from build123d import *

# Parameters (mm, degrees)
F1_DEPTH      = 16.002
F2_R          = 6.1442753349
F2_R_2        = 6.1243758279
F3_DEPTH      = 16.003
F5_DEPTH      = 25.4
F5_DEPTH_BACK = 25.4
F7_DEPTH      = 24.13
F7_DEPTH_BACK = 27.178
F8_R          = 3.5427392295
F9_DEPTH      = 25.4
F9_DEPTH_BACK = 25.4


with BuildPart() as f1:
    # F0 (on Top) → F1 (new body)
    with BuildSketch(Plane.XY):
        with BuildLine():
            Line((-13.3363356008, 47.4925674498), (13.3363356008, 47.4925674498))
            ThreePointArc((13.3363356008, 47.4925674498), (0, 60.8289030506), (-13.3363356008, 47.4925674498))
        make_face()
        with BuildLine():
            Line((13.3894772224, 47.4925674498), (13.3363356008, 47.4925674498))
            ThreePointArc((13.3363356008, 47.4925674498), (0, 34.156231849), (-13.3363356008, 47.4925674498))
            Line((-13.3363356008, 47.4925674498), (-13.3363356008, -46.5860655079))
            ThreePointArc((-13.3363356008, -46.5860655079), (0.5964639692, -34.4016239833), (13.3894772224, -47.7778092027))
            Line((13.3894772224, -47.7778092027), (13.3894772224, 47.4925674498))
        make_face()
        with BuildLine():
            ThreePointArc((-13.3363356008, 47.4925674498), (0, 34.156231849), (13.3363356008, 47.4925674498))
            Line((13.3363356008, 47.4925674498), (-13.3363356008, 47.4925674498))
        make_face()
        with BuildLine():
            Line((-13.3363356008, -47.7778092027), (-13.3363356008, -46.5860655079))
            ThreePointArc((-13.3363356008, -46.5860655079), (-0.5964639692, -61.1539944221), (13.3894772224, -47.7778092027))
            Line((13.3894772224, -47.7778092027), (-13.3363356008, -47.7778092027))
        make_face()
        with BuildLine():
            ThreePointArc((13.3894772224, -47.7778092027), (0.5964639692, -34.4016239833), (-13.3363356008, -46.5860655079))
            Line((-13.3363356008, -46.5860655079), (-13.3363356008, -47.7778092027))
            Line((-13.3363356008, -47.7778092027), (13.3894772224, -47.7778092027))
        make_face()
    extrude(amount=F1_DEPTH)

    # F2 (on Top) → F3 (cut, through all)
    with BuildSketch(Plane.XY):
        with Locations((0, 44.9254028499)):
            Circle(F2_R)
        with Locations((0, -46.6368459165)):
            Circle(F2_R_2)
    extrude(amount=F3_DEPTH, mode=Mode.SUBTRACT)

    # F4 (on Front) → F5 (join, two sides)
    with BuildSketch(Plane.XZ) as f5_sk:
        with BuildLine():
            ThreePointArc((6.5605365671, 36.938665784), (6.6343469805, 37.5070254574), (6.6590113547, 38.0796268582))
            ThreePointArc((6.6590113547, 38.0796268582), (0, 44.7386382129), (-6.6590113547, 38.0796268582))
            Line((-6.6590113547, 38.0796268582), (6.5605365671, 38.0796268582))
            Line((6.5605365671, 38.0796268582), (6.5605365671, 36.938665784))
        make_face()
        with BuildLine():
            Line((6.5605365671, 38.0796268582), (-6.6590113547, 38.0796268582))
            ThreePointArc((-6.6590113547, 38.0796268582), (-0.5726014008, 31.4452798778), (6.5605365671, 36.938665784))
            Line((6.5605365671, 36.938665784), (6.5605365671, 38.0796268582))
        make_face()
        with BuildLine():
            ThreePointArc((6.5605365671, 36.938665784), (-0.5726014008, 31.4452798778), (-6.6590113547, 38.0796268582))
            Line((-6.6590113547, 38.0796268582), (-6.6590113547, 2.7097861748))
            Line((-6.6590113547, 2.7097861748), (6.5605365671, 2.7097861748))
            Line((6.5605365671, 2.7097861748), (6.5605365671, 36.938665784))
        make_face()
    extrude(amount=F5_DEPTH)
    extrude(f5_sk.sketch, amount=-F5_DEPTH_BACK)

    # F6 (on Right) → F7 (cut, two sides)
    with BuildSketch(Plane.YZ) as f7_sk:
        with BuildLine():
            Line((6.0519274602, 27.9823391251), (6.0519274602, 27.4877400585))
            ThreePointArc((6.0519274602, 27.4877400585), (6.0557152675, 27.6113640409), (6.0569780455, 27.7350395918))
            ThreePointArc((6.0569780455, 27.7350395918), (6.0557152675, 27.8587151427), (6.0519274602, 27.9823391251))
        make_face()
        with BuildLine():
            Line((-6.0569780165, 27.7344470214), (6.0519274602, 27.4877400585))
            Line((6.0519274602, 27.4877400585), (6.0519274602, 27.9823391251))
            ThreePointArc((6.0519274602, 27.9823391251), (-0.1239717742, 33.7907488023), (-6.0569780165, 27.7344470214))
        make_face()
        with BuildLine():
            ThreePointArc((-6.0569780165, 27.7344470214), (-0.1233793273, 21.6793182817), (6.0519274602, 27.4877400585))
            Line((6.0519274602, 27.4877400585), (-6.0569780165, 27.7344470214))
        make_face()
        with BuildLine():
            Line((-6.08606264, 27.7350395918), (-6.0569780165, 27.7344470214))
            ThreePointArc((-6.0569780165, 27.7344470214), (-0.1239717742, 33.7907488023), (6.0519274602, 27.9823391251))
            Line((6.0519274602, 27.9823391251), (6.0519274602, 48.8666966558))
            Line((6.0519274602, 48.8666966558), (-6.08606264, 48.8666966558))
            Line((-6.08606264, 48.8666966558), (-6.08606264, 27.7350395918))
        make_face()
    extrude(amount=-F7_DEPTH, mode=Mode.SUBTRACT)
    extrude(f7_sk.sketch, amount=F7_DEPTH_BACK, mode=Mode.SUBTRACT)

    # F8 (on Front) → F9 (cut, two sides)
    with BuildSketch(Plane.XZ) as f9_sk:
        with Locations((0, 38.7586243451)):
            Circle(F8_R)
    extrude(amount=-F9_DEPTH, mode=Mode.SUBTRACT)
    extrude(f9_sk.sketch, amount=F9_DEPTH_BACK, mode=Mode.SUBTRACT)


solid = f1.part
Model file for the job. Use its own axes, mm. A direction names the side the tool comes from. Give positions to 0.01 mm unless a question says otherwise; leave off trailing zeros. Order: outer loops, then holes, each group sorted by start corner. A loop starts at its lowest first (then second) coordinate and runs counter-clockwise, first axis right, second up. Notation, with made-up numbers: (-9, 2.25) - (35, 2.25) arc R19 ccw to (35, 13.25) - close; hole circle Ø4 at (27.5, -5.5). An arc over 180 degrees is marked (long way). Write item = value, one per line. Start each with the question number.
1. Cut at D-D, the plane y = 0. List the corners of the cut face in (x, z).
2. Drop flat-ended pins along their axis: P1, Ø6.5, axis at y = 0, z = 26.5, coming from the +X side; P2, Ø4, axis at x = -2.5, z = 32.5, coming from the -Y side; P3, Ø6, axis at x = -1.5, y = -30.5, coming from the +Z side; P4, Ø5, axis at x = -1, z = 13.5, coming from the -Y side. Give the stop position or say it passes through.
3. Probe line 1 along Y through (x, z) = (0, 11.75); line 2 along Z through (x, y) = (0, 12.5); line 3 along Y through (x, z) = (5, 33). List the from-to ranges inside material, lowest first.
4. Cut at A-A, the plane x = 0. State how many separate pieces and enclosed holes the cut face has, and give its area (3 significant figures).
5. Cut at B-B, the plane z = 26. List the corners of the cut face in (x, y), and give its area (3 significant figures).
6. Two-plate mould, pull along Y, no slides. Class faces 1 (the flat face through (-6.659, -6, 25)), 2 (the cylindrical face through (0.293, 60.826, 7.889)), 3 (the flat face through (0, 6.052, 34)), 4 (the flat face through (0, -6.086, 34)): pulls with the +Y half, pulls with the -Y half, needs draft (parallel to the pull), parting line crosses it, or undercut.
7. Cut at C-C, the plane y = 20.5. List the corners of the cut face in (x, z).
8. Which spindle directions (+Z, -Z, +X, -X, +Y, -Y) get a long thin tool onto all of the face, cutting with end or side? Do faces 5 (the flat face through (0, -25.4, 27)), 6 (the flat face through (0, 25.4, 27)), 7 (the flat face through (6.561, -6, 26)). Say none if no direction does.
Taken from the geometry:
q1.outline = (-13.34, 0) - (13.39, 0) - (13.39, 16) - (6.56, 16) - (6.56, 21.68) - (-6.66, 21.68) - (-6.66, 16) - (-13.34, 16) - close
q2.P1 = through
q2.P2 = -25.4
q2.P3 = 16
q2.P4 = -61.17
q3.line_1 = -61.17 to -52.76, -40.51 to 38.78, 51.07 to 60.83
q3.line_2 = 0 to 35.22, 42.3 to 44.74
q3.line_3 = -25.4 to -6.09, 6.05 to 25.4
q4.separate_pieces = 5
q4.enclosed_holes = 0
q4.area = 2,480 mm²
q5.outline = (-6.66, -25.4) - (6.56, -25.4) - (6.56, -5.8) - (-6.66, -5.8) - close; (-6.66, 5.8) - (6.56, 5.8) - (6.56, 25.4) - (-6.66, 25.4) - close
q5.area = 518 mm²
q6.face_1 = needs draft
q6.face_2 = pulls with the +Y half
q6.face_3 = undercut
q6.face_4 = undercut
q7.outline = (-13.34, 0) - (13.39, 0) - (13.39, 16) - (6.56, 16) - (6.56, 36.94) arc R6.66 ccw (long way) to (-6.66, 38.08) - (-6.66, 16) - (-13.34, 16) - close; hole circle Ø7.09 at (0, 38.76)
q8.face_5 = +Z, +X, -X, -Y
q8.face_6 = +Z, +X, -X, +Y
q8.face_7 = +X, +Y, -Y
